```python
from build123d import *

# Parameters (mm, degrees)
F1_DEPTH = 2


with BuildPart() as f1:
    # F0 (on Top) → F1 (new body)
    with BuildSketch(Plane.XY):
        with BuildLine():
            ThreePointArc((-4.5, 12.196311), (-7.433034, -10.665365), (13, 0))
            ThreePointArc((13, 0), (10.665365, 7.433034), (4.5, 12.196311))
            ThreePointArc((4.5, 12.196311), (0, 13), (-4.5, 12.196311))
        make_face()
        with BuildLine():
            ThreePointArc((-1.25, -7.90174), (-8, 0), (-1.25, 7.90174))
            Line((-1.25, 7.90174), (-1.25, 5.40174))
            Line((-1.25, 5.40174), (1.25, 5.40174))
            Line((1.25, 5.40174), (1.25, 7.90174))
            ThreePointArc((1.25, 7.90174), (8, 0), (1.25, -7.90174))
            Line((1.25, -7.90174), (1.25, -5.40174))
            Line((1.25, -5.40174), (-1.25, -5.40174))
            Line((-1.25, -5.40174), (-1.25, -7.90174))
        make_face(mode=Mode.SUBTRACT)
        with BuildLine():
            ThreePointArc((-4.5, 12.196311), (0, 13), (4.5, 12.196311))
            Line((4.5, 12.196311), (6, 16.439282))
            ThreePointArc((6, 16.439282), (0, 17.5), (-6, 16.439282))
            Line((-6, 16.439282), (-4.5, 12.196311))
        make_face()
    extrude(amount=F1_DEPTH)


solid = f1.part
```
Geometry: final body of the model. Coordinates: model frame, mm. A direction names the side the tool comes from. Give positions to 0.01 mm unless a question says otherwise; leave off trailing zeros. Order: outer loops, then holes, each group sorted by start corner. A loop starts at its lowest first (then second) coordinate and runs counter-clockwise, first axis right, second up. Notation, with made-up numbers: M 85,-27.75 L 130,-27.75 A20 ccw 130,-7.75 Z; hole C 66,-0.75 d11. An arc over 180 degrees is marked long. Answer as CSV lines item,"result". Start each with the question number.
1) Cut plane A-A (x = 0). Output: boundary loops of the cut face in (y, z), then the cut area to 3 significant figures.
2) Cut plane B-B (z = 1.25). Output: boundary loops of the cut face in (x, y), then the cut area to 3 significant figures.
3) Cut plane C-C (y = -1.5). Output: boundary loops of the cut face in (x, z).
4) First-contact query: P1, Ø6, axis at x = 9.5, y = 3.5, coming from the -Z side; P2, Ø0.6, axis at y = 7, z = 1, coming from the +X side; P3, Ø0.6, axis at y = 7, z = 0.5, coming from the -X side; P4, Ø1, axis at y = -6, z = 1.5, coming from the +X side. Flat tips, straight axial feed; report the tip coordinate or a pass-through.
5) Cut plane D-D (y = 14). Output: boundary loops of the cut face in (x, z), then the cut area to 3 significant figures.
6) Line query: line 1 (X direction, y = -6, z = 1.25); line 2 (X direction, y = -4, z = 0.4); line 3 (X direction, y = 5, z = 0.55) (3 decimals). Output: solid intervals per line, ascending. Write a range as from..to.
7) Set-up query: faces 5 (the flat face through (5.24, 14.29, 0.99)), 6 (the flat face through (-5.26, 14.35, 0.99)), 7 (the flat face through (0, -5.402, 1)). Return all of +Z, -Z, +X, -X, +Y, -Y with unobstructed straight access to the full face (end or side cutting, diameter ignored); none if empty.
8) Mould query, pull axis Y, two halves, no side actions, for faces 1 (the flat face through (0, 5.402, 1)), 2 (the cylindrical face through (0.1, 17.5, 1)), 3 (the flat face through (0, 6, 0)), 4 (the flat face through (1.25, 7, 1)). Classes: +Y half, -Y half, draft (parallel to the pull), parting line (faces both ways), or undercut.
Findings below:
1,outline,"M -13,0 L -5.4,0 L -5.4,2 L -13,2 Z; M 5.4,0 L 17.5,0 L 17.5,2 L 5.4,2 Z"
1,area,"39.4 mm²"
2,outline,"M -6,16.44 L -4.5,12.2 A13 ccw long 4.5,12.2 L 6,16.44 A17.5 ccw Z; hole M -1.25,-7.9 L -1.25,-5.4 L 1.25,-5.4 L 1.25,-7.9 A8 ccw 1.25,7.9 L 1.25,5.4 L -1.25,5.4 L -1.25,7.9 A8 ccw Z"
2,area,"391 mm²"
3,outline,"M -12.91,0 L -7.86,0 L -7.86,2 L -12.91,2 Z; M 7.86,0 L 12.91,0 L 12.91,2 L 7.86,2 Z"
4,P1,"stops at z = 0"
4,P2,"stops at x = 11.14"
4,P3,"stops at x = -11.14"
4,P4,"stops at x = 11.78"
5,outline,"M -5.14,0 L 5.14,0 L 5.14,2 L -5.14,2 Z"
5,area,"20.6 mm²"
6,line 1,"x = -11.53..-5.29, -1.25..1.25, 5.29..11.53"
6,line 2,"x = -12.37..-6.93, 6.93..12.37"
6,line 3,"x = -12..-6.245, 6.245..12"
7,face 5,"+Z, -Z, +X"
7,face 6,"+Z, -Z, -X"
7,face 7,"+Z, -Z"
8,face 1,"undercut"
8,face 2,"+Y half"
8,face 3,"draft"
8,face 4,"undercut"
